Part model, mm, in its own coordinate system. A direction names the side the tool comes from. Round coordinates to 2 decimals unless told otherwise and drop trailing zeros. Loops run counter-clockwise (first coordinate to the right, second up) from the corner with the lowest first, then second, coordinate; pieces in that order, holes last. Notation, with made-up numbers: (-26, 61.25) - (17, 61.25) arc R26 ccw to (17, 80.25) - close; hole circle Ø4 at (74, 6). An arc over 180 degrees is marked (long way). Put each result on its own line as item: value.
from build123d import *

# Parameters (mm, degrees)
F0_W     = 117.9269552231
F0_H     = 117.9269552231
F0_R     = 15.0136724475
F0_R_2   = 5.0045574825
F1_DEPTH = 50
F2_DEPTH = 137.4
F3_R     = 9.6568542495
F5_R     = 16.8994949366
F6_SIZE  = 20


# Not quite as in the source:
# - a fillet or chamfer that OpenCascade refuses, or shapes differently, is made with other operations: its cross-section is extruded or revolved along the edge and cut away or added


with BuildPart() as f1:
    # F0 (on Top) → F1 (new body)
    with BuildSketch(Plane.XY):
        Rectangle(F0_W, F0_H)
        Circle(F0_R, mode=Mode.SUBTRACT)
        Circle(F0_R)
        Circle(F0_R_2, mode=Mode.SUBTRACT)
    extrude(amount=F1_DEPTH)

    # F0 (on Top) → F2 (join)
    with BuildSketch(Plane.XY):
        Circle(F0_R)
        Circle(F0_R_2, mode=Mode.SUBTRACT)
    extrude(amount=F2_DEPTH)

    # F3
    f3_edges = [f1.edges().sort_by_distance(p)[0] for p in [
        (-15.013672, 0, 137.4),
    ]]
    fillet(f3_edges, radius=F3_R)

    # F4: chamfer of 5 on 1 edges, made by hand

    # F4_s1 → F4_t2 (revolve, cut)
    with BuildSketch(Plane.XZ):
        Polygon((10.0045574825, 137.4), (5.0045574825, 132.4), (5.0045574825, 137.4), align=None)
    revolve(axis=Axis((0, 0, 137.4), (0, 0, 1)), mode=Mode.SUBTRACT)

    # F5
    f5_edges = [f1.edges().sort_by_distance(p)[0] for p in [
        (58.963478, 0, 50),
        (0, -58.963478, 50),
        (0, 58.963478, 50),
        (-58.963478, 0, 50),
        (-15.013672, 0, 50),
    ]]
    fillet(f5_edges, radius=F5_R)

    # F6
    f6_edges = [f1.edges().sort_by_distance(p)[0] for p in [
        (-58.963478, 0, 0),
        (0, 58.963478, 0),
        (58.963478, 0, 0),
        (0, -58.963478, 0),
        (-5.004557, 0, 0),
    ]]
    chamfer(f6_edges, length=F6_SIZE)


solid = f1.part
1. Band-saw the part on D-D (z = 15.5). List the corners of the cut face in (x, y), plus the area to 3 significant figures.
A:
outline: (-54.46, -54.46) - (54.46, -54.46) - (54.46, 54.46) - (-54.46, 54.46) - close; hole circle Ø19.01 at (0, 0)
area: 11,600 mm²
2. Probe line 1 along Y through (x, z) = (0, 107.5); line 2 along Y through (x, z) = (29, 34); line 3 along Y through (x, z) = (0, 59). List the from-to ranges inside material, lowest first. Write a range as [from, to].
A:
line 1: y = [-15.01, -5], [5, 15.01]
line 2: y = [-58.94, 58.94]
line 3: y = [-16.97, -5], [5, 16.97]
3. Tool access for faces 5 (the cylindrical face through (-11.066, 10.147, 96.895)), 6 (the cylindrical face through (-3.69, 3.38, 75.41)): list every direction of +Z, -Z, +X, -X, +Y, -Y with a clear straight run to the whole face (end or side of a thin tool).
A:
face 5: +Z
face 6: +Z, -Z
4. Band-saw the part on B-B (z = 110.5). List the corners of the cut face in (x, y), plus the area to 3 significant figures.
A:
outline: circle Ø30.03 at (0, 0); hole circle Ø10.01 at (0, 0)
area: 629 mm²
5. Band-saw the part on C-C (y = 50.5). List the corners of the cut face in (x, z), plus the area to 3 significant figures.
A:
outline: (-58.96, 20) - (-50.5, 11.54) - (50.5, 11.54) - (58.96, 20) - (58.96, 33.1) arc R16.9 ccw to (50.5, 47.74) - (-50.5, 47.74) arc R16.9 ccw to (-58.96, 33.1) - close
area: 4,130 mm²
6. Band-saw the part on A-A (x = -34). List the corners of the cut face in (y, z), plus the area to 3 significant figures.
A:
outline: (-58.96, 20) - (-38.96, 0) - (38.96, 0) - (58.96, 20) - (58.96, 33.1) arc R16.9 ccw to (42.06, 50) - (-42.06, 50) arc R16.9 ccw to (-58.96, 33.1) - close
area: 5,370 mm²
7. Two-plate mould, pull along Y, no slides. Class faces 1 (the flat face through (-0.825, 48.823, 9.86)), 2 (the conical face through (-1.838, -8.276, 16.527)), 3 (the flat face through (-0.825, -48.823, 9.86)), 4 (the cylindrical face through (-53.88, 0.83, 45.18)): pulls with the +Y half, pulls with the -Y half, needs draft (parallel to the pull), parting line crosses it, or undercut.
A:
face 1: pulls with the +Y half
face 2: undercut
face 3: pulls with the -Y half
face 4: needs draft
8. Pin check, flat tips, straight feed: P1, Ø3, axis at x = -41.5, y = -8.5, coming from the -Z side; P2, Ø3, axis at y = 1, z = 116.5, coming from the +X side; P3, Ø13, axis at x = 0, y = 0, coming from the -Z side. Stop position of each tip, or through.
A:
P1: stops at z = 1.04
P2: stops at x = 15.01
P3: stops at z = 18.5
